Check sheet for the modelled part. Datum: model origin and axes. Units: mm. A direction names the side the tool comes from. Coordinates: 2 decimals unless noted, no trailing zeros. Order: outer loops, then holes, each group sorted by start corner. A loop starts at its lowest first (then second) coordinate and runs counter-clockwise, first axis right, second up.
1. Cross-section at A-A (y = 140). Enter the section's corners in (x, z).
2. Cross-section at D-D (y = 85). Enter the section's corners in (x, z), then the cut area to 3 significant figures.
3. Cross-section at C-C (x = 17.5). Enter the section's corners in (y, z), then the cut area to 4 significant figures.
4. Cross-section at B-B (z = -9). Enter the section's corners in (x, y).
5. Set-up check for faces 4 (the flat face through (20, 22, 0)), 5 (the flat face through (-38, 90, 20)), 6 (the flat face through (37, 170, 0)), 7 (the flat face through (-38, 90, -20)), 8 (the flat face through (-24, 18, -2.5)): record each of +Z, -Z, +X, -X, +Y, -Y from which the full face is reachable in a straight line by a thin tool's end or side.
6. Gauge pin test, flat ends, axial feed: pin 1 Ø10 at (x, y) = (24, 22.5) entering from +Z; pin 2 Ø12 at (x, y) = (-40.5, 118.5) entering from -Z; pin 3 Ø1.5 at (x, y) = (-27.5, 99.5) entering from +Z; pin 4 Ø1 at (x, z) = (25, -6) entering from +Y. Record the tip position at first contact, or that the pin passes through.
7. Thickness scan on line 1 (Y direction, x = -34.5, z = 0); line 2 (X direction, y = 67, z = -5); line 3 (X direction, y = 6, z = 0). Record the ranges inside material, lowest first.
8. Draft check along Z on faces 1 (the cylindrical face through (37.4, 135.12, 1.08)), 2 (the flat face through (37, 90, 20)), 3 (the flat face through (24, 18, -2.5)). Enter one of: released by +Z, released by -Z, zero draft, split by the parting line, or undercut.
```python
from build123d import *

# Parameters (mm, degrees)
SKETCH_1_W               = 90
SKETCH_1_H               = 80
EXTRUDE_1_DEPTH          = 12
SKETCH_2_W               = 15
SKETCH_2_H               = 40
EXTRUDE_2_DEPTH          = 158
CUT_EXTRUDE_1_DEPTH      = 181.346887969
CUT_EXTRUDE_1_DEPTH_BACK = 181.346887969
SKETCH_3_R               = 5
CUT_EXTRUDE_2_DEPTH      = 170.082819943
CUT_EXTRUDE_2_DEPTH_BACK = 10
SKETCH_4_R               = 1.25
RIB_6_REACH              = 182.347
SKETCH_6_WALL_W          = 28.284271248
SKETCH_6_WALL_H          = 5


with BuildPart() as part:
    # 草图1 → 凸台-拉伸1 (new body)
    with BuildSketch(Plane(origin=(0, 0, 0), x_dir=(1, 0, 0), z_dir=(0, 1, 0))):
        Rectangle(SKETCH_1_W, SKETCH_1_H)
    extrude(amount=EXTRUDE_1_DEPTH)

    # 草图2 → 凸台-拉伸2 (add)
    with BuildSketch(Plane(origin=(0, 12, 0), x_dir=(1, 0, 0), z_dir=(0, 1, 0))):
        with Locations((-37.5, 0)):
            Rectangle(SKETCH_2_W, SKETCH_2_H)
        with Locations((37.5, 0)):
            Rectangle(SKETCH_2_W, SKETCH_2_H)
    extrude(amount=EXTRUDE_2_DEPTH)

    # 草图3 → 切除-拉伸1 (cut, two sides: drawn at the far end of the back side and taken through both)
    with BuildSketch(Plane(origin=(0, 0, 0), x_dir=(0, 0, -1), z_dir=(1, 0, 0)).offset(-CUT_EXTRUDE_1_DEPTH_BACK)):
        with Locations((0, 140)):
            Circle(SKETCH_3_R)
    extrude(amount=CUT_EXTRUDE_1_DEPTH + CUT_EXTRUDE_1_DEPTH_BACK, mode=Mode.SUBTRACT)

    # 草图4 → 切除-拉伸2 (cut, two sides: drawn at the far end of the back side and taken through both)
    with BuildSketch(Plane(origin=(0, 12, 0), x_dir=(1, 0, 0), z_dir=(0, 1, 0)).offset(-CUT_EXTRUDE_2_DEPTH_BACK)):
        with Locations(Location((0, 0, 0), (0, 0, 270))):
            Circle(SKETCH_4_R)
    extrude(amount=CUT_EXTRUDE_2_DEPTH + CUT_EXTRUDE_2_DEPTH_BACK, mode=Mode.SUBTRACT)

    # 草图6 wall → 筋6 (add, up to next)
    with BuildSketch(Plane(origin=(-20, 22, 0), x_dir=(0.707106781187, -0.707106781187, 0), z_dir=(0.707106781187, 0.707106781187, 0)), mode=Mode.PRIVATE) as rib_6_sk1:
        Rectangle(SKETCH_6_WALL_W, SKETCH_6_WALL_H)
    rib_6_tool1 = extrude(rib_6_sk1.sketch, amount=-RIB_6_REACH, mode=Mode.PRIVATE) - part.part
    rib_6 = rib_6_tool1.solids().sort_by_distance((-20, 22, 0))[0]
    add(rib_6)

    # 镜向1: 筋6 across plane
    add(rib_6.mirror(Plane(origin=(0, 0, 0), x_dir=(0, 0, 1), z_dir=(1, 0, 0))))


solid = part.part
```
Data:
1. outline: (-45, -20) - (-30, -20) - (-30, -5) - (-45, -5) - close; (-45, 5) - (-30, 5) - (-30, 20) - (-45, 20) - close; (30, -20) - (45, -20) - (45, -5) - (30, -5) - close; (30, 5) - (45, 5) - (45, 20) - (30, 20) - close
2. outline: (-45, -20) - (-30, -20) - (-30, 20) - (-45, 20) - close; (30, -20) - (45, -20) - (45, 20) - (30, 20) - close
2. area: 1,200 mm2
3. outline: (0, -40) - (12, -40) - (12, -2.5) - (19.5, -2.5) - (19.5, 2.5) - (12, 2.5) - (12, 40) - (0, 40) - close
3. area: 997.5 mm2
4. outline: (-45, 0) - (45, 0) - (45, 170) - (30, 170) - (30, 12) - (-30, 12) - (-30, 170) - (-45, 170) - close
5. face 4: +Z, -Z, +Y
5. face 5: +Z, +X, -X, +Y
5. face 6: +Z, -Z, +X, -X, +Y
5. face 7: -Z, +X, -X, +Y
5. face 8: -Z, +Y
6. pin 1: stops at z = 2.5
6. pin 2: stops at z = -20
6. pin 3: passes through
6. pin 4: stops at y = 12
7. line 1: y = 0 to 135, 145 to 170
7. line 2: x = -45 to -30, 30 to 45
7. line 3: x = -45 to -1.25, 1.25 to 45
8. face 1: undercut
8. face 2: released by +Z
8. face 3: released by -Z
